Could you check a few things on this drawing? It's one solid part, dimensions in mm from its lowest x, y, z. Give positions to 0.01 mm unless a question says otherwise; leave off trailing zeros. Loops run counter-clockwise (first coordinate to the right, second up) from the corner with the lowest first, then second, coordinate; pieces in that order, holes last. Notation, with made-up numbers: M -13,15.25 L 29,15.25 A15 cw 29,32.25 Z; hole C 2.25,40 d9. An arc over 180 degrees is marked long. Answer as CSV lines item,"result". Start each with the question number.
Item 1: I want a section at A-A on y = 5. List the corners of the cut face in (x, z) for me.
Item 2: Will this pin go through, and if not, where does the flat tip stop? P1, Ø4, axis at y = 32.79, z = 17.91, coming from the -X side.
Item 3: I want a section at B-B on x = 10. Give the number of separate pieces and of enclosed holes in the cut face, plus the area to 3 significant figures.
Item 4: I want a section at C-C on z = 12.5. List the corners of the cut face in (x, y) for me.
Item 5: If we mould it in two halves opening along Y, with no side actions, what happens to the marked faces 1, 2 and 3? For each: released by +Y, released by -Y, zero draft, split by the parting line, or undercut.
Item 6: If I drill on line 1 along Z through (x, y) = (9, 25); line 2 along Y through (x, z) = (17.5, 18) (1 decimal); line 3 along Y through (x, z) = (8.25, 13.25), over which ranges is the centre line in solid material (lowest first)? Write a range as from..to.
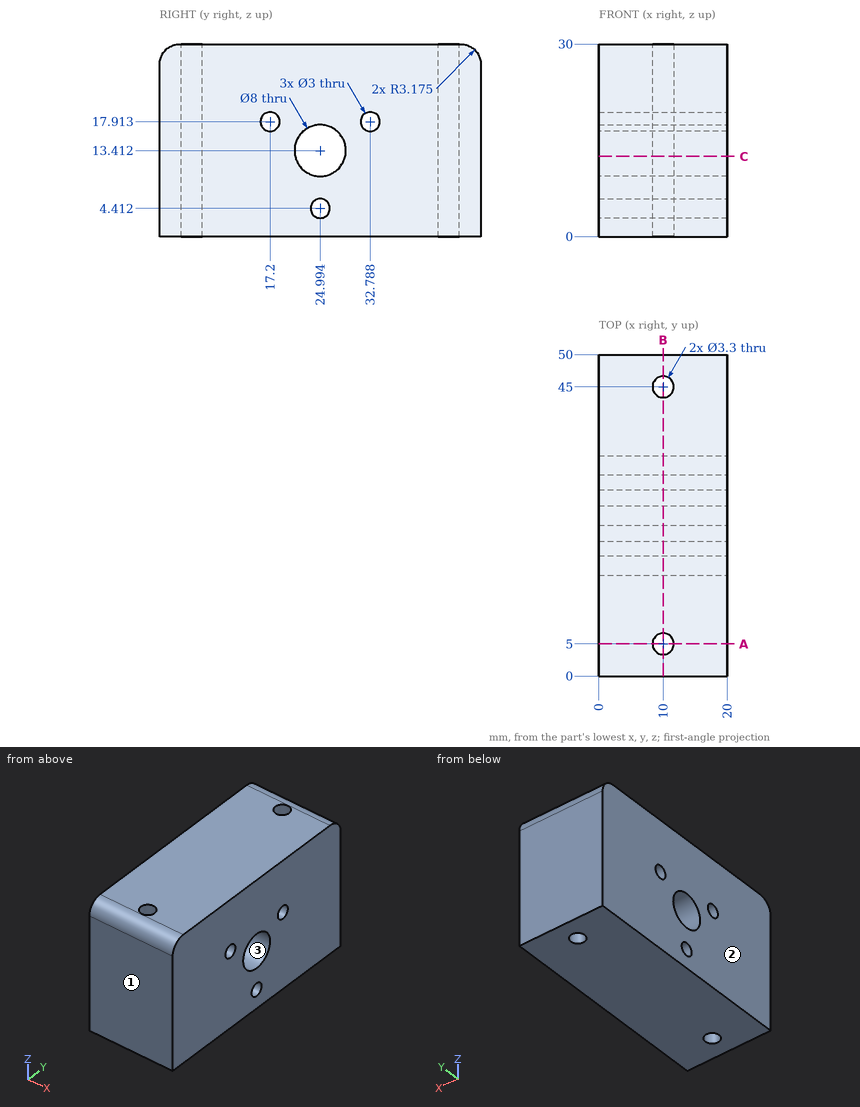
Result:
1,outline,"M 0,0 L 8.35,0 L 8.35,30 L 0,30 Z; M 11.65,0 L 20,0 L 20,30 L 11.65,30 Z"
2,P1,"x = 0"
3,separate pieces,"3"
3,enclosed holes,"4"
3,area,"1,230 mm^2"
4,outline,"M 0,0 L 20,0 L 20,21.1 L 0,21.1 Z; M 0,28.89 L 20,28.89 L 20,50 L 0,50 Z; hole C 10,5 d3.3; hole C 10,45 d3.3"
5,face 1,"released by -Y"
5,face 2,"zero draft"
5,face 3,"undercut"
6,line 1,"0..2.91, 5.91..9.41, 17.41..30"
6,line 2,"0..15.7, 18.7..31.3, 34.3..50"
6,line 3,"0..21, 28.99..50"
